from build123d import *

# Parameters (mm, degrees)
BOSS_EXTRUDE1_DEPTH             = 12
CUT_EXTRUDE1_DEPTH              = 26.760554208
SKETCH4_R                       = 4.75
SKETCH4_R_2                     = 1.25
BOSS_EXTRUDE2_DEPTH             = 1.5
BOSS_EXTRUDE2_DIRECTION_2_REACH = 28.092
BOSS_EXTRUDE3_START             = -5
BOSS_EXTRUDE3_OUTLINE_R         = 1.25
BOSS_EXTRUDE3_DEPTH             = 5
SKETCH6_R                       = 0.95
CUT_EXTRUDE2_DEPTH              = 3
BOSS_EXTRUDE4_START             = -1
SKETCH8_R                       = 1.25
SKETCH8_R_2                     = 0.79375
BOSS_EXTRUDE4_DEPTH             = 1
BOSS_EXTRUDE5_DEPTH             = 0.625
SKETCH11_R                      = 1.532291667
BOSS_EXTRUDE6_DEPTH             = 3.175
CUT_EXTRUDE3_DEPTH              = 1.5875
SKETCH13_R                      = 1.532291667
BOSS_EXTRUDE7_DEPTH             = 1.5875
CUT_EXTRUDE4_DEPTH              = 1.5875


# Read off the part's stored shape, not the designer's step: Boss-Extrude3
with BuildPart() as part:
    # Sketch1 → Boss-Extrude1 (new body)
    with BuildSketch(Plane.XY):
        with BuildLine():
            Line((-1.765801731, 4.94680722), (-7.765801731, 4.94680722))
            Line((-7.765801731, 4.94680722), (-7.765801731, 2.16867722))
            Line((-7.765801731, 2.16867722), (-2.421629262, 2.16867722))
            Line((-2.421629262, 2.16867722), (2.456068269, -0.270171545))
            Line((2.456068269, -0.270171545), (2.456068269, -10.53131278))
            ThreePointArc((2.456068269, -10.53131278), (4.06858061, -10.971275495), (5.234198269, -12.169231551))
            Line((5.234198269, -12.169231551), (5.234198269, 1.44680722))
            Line((5.234198269, 1.44680722), (-1.765801731, 4.94680722))
        make_face()
        with BuildLine():
            Line((5.234198269, -15.243394008), (5.234198269, -12.169231551))
            ThreePointArc((5.234198269, -12.169231551), (4.06858061, -10.971275495), (2.456068269, -10.53131278))
            Line((2.456068269, -10.53131278), (2.456068269, -12.51568778))
            ThreePointArc((2.456068269, -12.51568778), (3.29796728, -12.864413768), (3.646693269, -13.70631278))
            ThreePointArc((3.646693269, -13.70631278), (2.456068269, -14.89693778), (1.265443269, -13.70631278))
            Line((1.265443269, -13.70631278), (-0.718931731, -13.70631278))
            ThreePointArc((-0.718931731, -13.70631278), (-0.278969016, -15.318825121), (0.91898704, -16.48444278))
            Line((0.91898704, -16.48444278), (3.993149497, -16.48444278))
            ThreePointArc((3.993149497, -16.48444278), (4.701132299, -15.95137681), (5.234198269, -15.243394008))
        make_face()
        with BuildLine():
            Line((2.456068269, -12.51568778), (2.456068269, -10.53131278))
            ThreePointArc((2.456068269, -10.53131278), (0.211004238, -11.461248749), (-0.718931731, -13.70631278))
            Line((-0.718931731, -13.70631278), (1.265443269, -13.70631278))
            ThreePointArc((1.265443269, -13.70631278), (1.614169257, -12.864413768), (2.456068269, -12.51568778))
        make_face()
        with BuildLine():
            ThreePointArc((5.631068269, -13.70631278), (5.530250091, -12.91256778), (5.234198269, -12.169231551))
            Line((5.234198269, -12.169231551), (5.234198269, -15.243394008))
            ThreePointArc((5.234198269, -15.243394008), (5.530250091, -14.50005778), (5.631068269, -13.70631278))
        make_face()
        with BuildLine():
            ThreePointArc((0.91898704, -16.48444278), (2.456068269, -16.88131278), (3.993149497, -16.48444278))
            Line((3.993149497, -16.48444278), (0.91898704, -16.48444278))
        make_face()
        with BuildLine():
            ThreePointArc((0.91898704, -16.48444278), (-0.278969016, -15.318825121), (-0.718931731, -13.70631278))
            Line((-0.718931731, -13.70631278), (-7.765801731, -13.70631278))
            Line((-7.765801731, -13.70631278), (-7.765801731, -16.48444278))
            Line((-7.765801731, -16.48444278), (0.91898704, -16.48444278))
        make_face()
    extrude(amount=BOSS_EXTRUDE1_DEPTH)

    # Sketch3 → Cut-Extrude1 (cut, through all)
    with BuildSketch(Plane.XZ.offset(16.48444278)):
        Polygon((-7.765801731, 9.5), (-2.08101296, 12), (-7.765801731, 12), align=None)
    extrude(amount=-CUT_EXTRUDE1_DEPTH, mode=Mode.SUBTRACT)

    # Sketch4 → Boss-Extrude2 (add)
    with BuildSketch(Plane(origin=(0, 4.94680722, 0), x_dir=(1, 0, 0), z_dir=(0, 1, 0))):
        with Locations(Location((-9.515801731, -5.084119567, 0), (0, 0, 180))):
            Circle(SKETCH4_R)
        with Locations(Location((-9.515801731, -5.084119567, 0), (0, 0, 180))):
            Circle(SKETCH4_R_2, mode=Mode.SUBTRACT)
    extrude(amount=BOSS_EXTRUDE2_DEPTH)

    # Boss-Extrude2 direction 2: up to this face of the body (flat: up to its plane)
    boss_extrude2_direction_2_end = Plane(part.part.faces().sort_by_distance((-4.995668733, 2.16867722, 5.359110802))[0])
    # Sketch4 → Boss-Extrude2 direction 2 (add, up to the picked face)
    with BuildSketch(Plane(origin=(0, 4.94680722, 0), x_dir=(1, 0, 0), z_dir=(0, 1, 0)), mode=Mode.PRIVATE) as boss_extrude2_direction_2_sk1:
        with Locations(Location((-9.515801731, -5.084119567, 0), (0, 0, 180))):
            Circle(SKETCH4_R)
        with Locations(Location((-9.515801731, -5.084119567, 0), (0, 0, 180))):
            Circle(SKETCH4_R_2, mode=Mode.SUBTRACT)
    boss_extrude2_direction_2_tool1 = split(extrude(boss_extrude2_direction_2_sk1.sketch, amount=-BOSS_EXTRUDE2_DIRECTION_2_REACH, mode=Mode.PRIVATE), bisect_by=boss_extrude2_direction_2_end, keep=Keep.BOTH, mode=Mode.PRIVATE)
    add(boss_extrude2_direction_2_tool1.solids().sort_by(Axis((-4.900152, 4.946807, 5.08412), (0, -1, 0)))[0])

    # Boss-Extrude3 outline → Boss-Extrude3 (add)
    with BuildSketch(Plane(origin=(0, -13.70631278, 0), x_dir=(1, 0, 0), z_dir=(0, 1, 0)).offset(BOSS_EXTRUDE3_START)):
        with BuildLine():
            ThreePointArc((-5.39824459, -2.715950825), (-14.265801731, -5.084119567), (-5.39824459, -7.452288309))
            Line((-5.39824459, -7.452288309), (-4.405194864, -5.725663462))
            ThreePointArc((-4.405194864, -5.725663462), (-4.233864229, -5.084119567), (-4.405194864, -4.442575672))
            Line((-4.405194864, -4.442575672), (-5.39824459, -2.715950825))
        make_face()
        with Locations((-9.515801731, -5.084119567)):
            Circle(BOSS_EXTRUDE3_OUTLINE_R, mode=Mode.SUBTRACT)
    extrude(amount=BOSS_EXTRUDE3_DEPTH)

    # Sketch6 → Cut-Extrude2 (cut)
    with BuildSketch(Plane.XZ.offset(18.70631278)):
        with Locations(Location((-6.24983298, 5.084119567, 0), (0, 0, 270))):
            Circle(SKETCH6_R)
    extrude(amount=-CUT_EXTRUDE2_DEPTH, mode=Mode.SUBTRACT)

    # Sketch8 → Boss-Extrude4 (add)
    with BuildSketch(Plane(origin=(0, 6.44680722, 0), x_dir=(1, 0, 0), z_dir=(0, 1, 0)).offset(BOSS_EXTRUDE4_START)):
        with Locations(Location((-9.515801731, -5.084119567, 0), (0, 0, 180))):
            Circle(SKETCH8_R)
        with Locations(Location((-9.515801731, -5.084119567, 0), (0, 0, 180))):
            Circle(SKETCH8_R_2, mode=Mode.SUBTRACT)
    extrude(amount=BOSS_EXTRUDE4_DEPTH)

    # Sketch9 → Boss-Extrude5 (add)
    with BuildSketch(Plane(origin=(0, 0, 2.38125), x_dir=(-1, 0, 0), z_dir=(0, 0, -1))):
        Polygon((5.971387176, 2.16867722), (-2.456068269, -2.045050502), (-2.456068269, -0.270171545), (2.421629262, 2.16867722), align=None)
        Polygon((4.642221382, -13.70631278), (-2.456068269, -10.156401543), (-2.456068269, -11.535790724), (0, -13.70631278), align=None)
    extrude(amount=-BOSS_EXTRUDE5_DEPTH)

    # Sketch11 → Boss-Extrude6 (add)
    with BuildSketch(Plane(origin=(0, 0, 1.5875), x_dir=(-1, 0, 0), z_dir=(0, 0, -1))):
        with BuildLine():
            Line((-5.234198269, 1.44680722), (-5.234198269, 9.827015554))
            ThreePointArc((-5.234198269, 9.827015554), (-4.320432445, 12.033041397), (-2.114406602, 12.94680722))
            Line((-2.114406602, 12.94680722), (5.602260065, 12.94680722))
            ThreePointArc((5.602260065, 12.94680722), (7.808285908, 12.033041397), (8.722051731, 9.827015554))
            Line((8.722051731, 9.827015554), (8.722051731, 6.44680722))
            Line((8.722051731, 6.44680722), (8.722051731, 4.94680722))
            Line((8.722051731, 4.94680722), (1.765801731, 4.94680722))
            Line((1.765801731, 4.94680722), (-5.234198269, 1.44680722))
        make_face()
        with Locations((5.602260065, 9.827015554)):
            Circle(SKETCH11_R, mode=Mode.SUBTRACT)
        with Locations((1.743926731, 9.827015554)):
            Circle(SKETCH11_R, mode=Mode.SUBTRACT)
        with Locations((-2.114406602, 9.827015554)):
            Circle(SKETCH11_R, mode=Mode.SUBTRACT)
    extrude(amount=-BOSS_EXTRUDE6_DEPTH)

    # Sketch14 → Cut-Extrude3 (cut)
    with BuildSketch(Plane.XY.offset(4.7625)):
        Polygon((3.634198269, 2.24680722), (3.634198269, 6.94680722), (-2.365801731, 6.94680722), (-2.365801731, 4.94680722), (-1.765801731, 4.94680722), align=None)
    extrude(amount=-CUT_EXTRUDE3_DEPTH, mode=Mode.SUBTRACT)

    # Sketch12 → Revolve1 (revolve)
    with BuildSketch(Plane(origin=(2.114406602, 0, 0), x_dir=(0, 0, -1), z_dir=(1, 0, 0)), mode=Mode.PRIVATE) as revolve1_sk:
        with BuildLine():
            Line((-6.7625, 10.827015554), (-7.2625, 10.827015554))
            ThreePointArc((-7.2625, 10.827015554), (-8.67222129, 11.800758233), (-10.31875, 11.327015554))
            Line((-10.31875, 11.327015554), (-10.31875, 9.827015554))
            Line((-10.31875, 9.827015554), (-1.5875, 9.827015554))
            Line((-1.5875, 9.827015554), (3.175, 9.827015554))
            Line((3.175, 9.827015554), (3.175, 11.35930722))
            Line((3.175, 11.35930722), (-1.5875, 11.35930722))
            Line((-1.5875, 11.35930722), (-4.7625, 11.35930722))
            Line((-4.7625, 11.35930722), (-4.7625, 12.605140554))
            Line((-4.7625, 12.605140554), (-5.55625, 12.605140554))
            Line((-5.55625, 12.605140554), (-6.7625, 10.827015554))
        make_face()
    revolve(revolve1_sk.sketch.rotate(Axis((2.114406602, 9.827015554, 4.7625), (0, 0, -1)), 90), axis=Axis((2.114406602, 9.827015554, 4.7625), (0, 0, -1)))

    # Sketch13 → Boss-Extrude7 (add)
    with BuildSketch(Plane(origin=(0, 0, 1.5875), x_dir=(-1, 0, 0), z_dir=(0, 0, -1))):
        Polygon((-0.130031602, 10.972694994), (-2.114406602, 12.118374435), (-4.098781602, 10.972694994), (-4.098781602, 8.681336113), (-2.114406602, 7.535656673), (-0.130031602, 8.681336113), align=None)
        with Locations(Location((-2.114406602, 9.827015554, 0), (0, 0, 180))):
            Circle(SKETCH13_R, mode=Mode.SUBTRACT)
    extrude(amount=BOSS_EXTRUDE7_DEPTH)

    # Sketch15 → Cut-Extrude4 (cut)
    with BuildSketch(Plane.XY.offset(10.31875)):
        Polygon((3.455328551, 9.827015554), (2.784867577, 10.988288026), (1.443945627, 10.988288026), (0.773484653, 9.827015554), (1.443945627, 8.665743081), (2.784867577, 8.665743081), align=None)
    extrude(amount=-CUT_EXTRUDE4_DEPTH, mode=Mode.SUBTRACT)


solid = part.part
Geometry: final body of the model. Coordinates: model frame, mm. A direction names the side the tool comes from. Give positions to 0.01 mm unless a question says otherwise; leave off trailing zeros. Loops run counter-clockwise (first coordinate to the right, second up) from the corner with the lowest first, then second, coordinate; pieces in that order, holes last. Notation, with made-up numbers: (50, 21.25) - (76, 21.25) arc R11 ccw to (76, 28.25) - close; hole circle Ø1 at (-0.75, 6). An arc over 180 degrees is marked (long way). Answer as CSV lines item,"result". Start each with the question number.
1. Section C-C, the plane y = -1. Return loops of the section in (x, z).
2. Draft query along Y for faces 1 (the face through (-7.78, 12.06, 3.15)), 2 (the face through (-8.722, 8, 3)), 3 (the face through (3.634, 5, 4)). Return one class per face: released by +Y, released by -Y, zero draft, split by the parting line, or undercut.
3. Pin query (flat end, axial travel): P1, Ø4, axis at x = -5.6, y = 9.83, coming from the +Z side; P2, Ø1, axis at x = -4.5, y = -15.5, coming from the +Z side; P3, Ø1.3, axis at x = 1, z = 4.5, coming from the -Y side. Return the tip coordinate at first contact, or that it passes through.
4. Section A-A, the plane x = -9.75. Return loops of the section in (y, z).
5. Ray query, L1, parallel to Y at x = -3.25, z = 0.5; L2, parallel to X at y = 10.5, z = 1.75; L3, parallel to Y at x = -9.75, z = 3.25. Return the intervals inside material, ascending.
6. Reachability of faces 4 (the face through (1.783, 3.172, 7.526)), 5 (the face through (-5, 4.947, 1)), 6 (the face through (0.13, 10, 1)), 7 (the face through (-1, 1, 3.006)) from +Z, -Z, +X, -X, +Y, -Y: full face, straight path, thin tool, end or side. Return the list, or none.
7. Section D-D, the plane y = 9.5. Give the number of separate pieces and of enclosed holes in the cut face, plus the area to 3 significant figures.
Answers:
1,outline,"(0.37, 2.38) - (2.46, 2.38) - (2.46, 0) - (5.23, 0) - (5.23, 12) - (2.46, 12) - (2.46, 3.01) - (0.37, 3.01) - close"
2,face 1,"released by +Y"
2,face 2,"zero draft"
2,face 3,"undercut"
3,P1,"stops at z = 4.76"
3,P2,"stops at z = 11.16"
3,P3,"stops at y = -16.78"
4,outline,"(-18.71, 0.34) - (-13.71, 0.34) - (-13.71, 3.86) - (-18.71, 3.86) - close; (-18.71, 6.31) - (-13.71, 6.31) - (-13.71, 9.83) - (-18.71, 9.83) - close; (2.17, 0.34) - (6.45, 0.34) - (6.45, 4.33) - (5.45, 4.33) - (5.45, 3.86) - (2.17, 3.86) - close; (2.17, 6.31) - (5.45, 6.31) - (5.45, 5.84) - (6.45, 5.84) - (6.45, 9.83) - (2.17, 9.83) - close"
5,L1,"y = -16.48 to -13.71, 2.17 to 4.95"
5,L2,"x = -8.65 to -6.98, -4.23 to -3.12, -0.37 to 5.16"
5,L3,"y = -18.71 to -13.71, 2.17 to 6.45"
6,face 4,"+Z"
6,face 5,"-Z, +X, +Y"
6,face 6,"-Z, -X, +Y"
6,face 7,"+Z, -X"
7,separate pieces,"3"
7,enclosed holes,"0"
7,area,"57.9 mm2"
